Geometry check sheet. Reference: drawing and pictorial views, mm from the part's lowest x, y, z. A direction names the side the tool comes from. Round coordinates to 2 decimals unless told otherwise and drop trailing zeros. Order: outer loops, then holes, each group sorted by start corner. A loop starts at its lowest first (then second) coordinate and runs counter-clockwise, first axis right, second up.
(1) Depth check by flat-ended pin: pin 1 (1 mm diameter, centred on y = 5, z = 5, fed in from +X); pin 2 (0.6 mm diameter, centred on x = 49.5, y = 6, fed in from +Z); pin 3 (2 mm diameter, centred on x = 52, z = 5.5, fed in from +Y). Enter the tip coordinate at first touch or a pass-through.
(2) Tool access check on the marked faces 1, 2 and 3. Record the directions out of +Z, -Z, +X, -X, +Y, -Y that give a thin tool (end or side, any length) a straight path to the whole face; none if there is none.
(3) Sectioned sample at B-B, the plane z = 4.2. Enter the section's corners in (x, y), and give its area (3 significant figures).
(4) Thickness scan on probe 1 along X at (y, z) = (1.75, 0.35); probe 2 along Z at (x, y) = (70, 0.5); probe 3 along Z at (x, y) = (44, 1.5). Record the ranges inside material, lowest first.
(5) Sectioned sample at A-A, the plane y = 3. Enter the section's corners in (x, z).
(6) Sectioned sample at C-C, the plane x = 66. Enter the section's corners in (y, z).
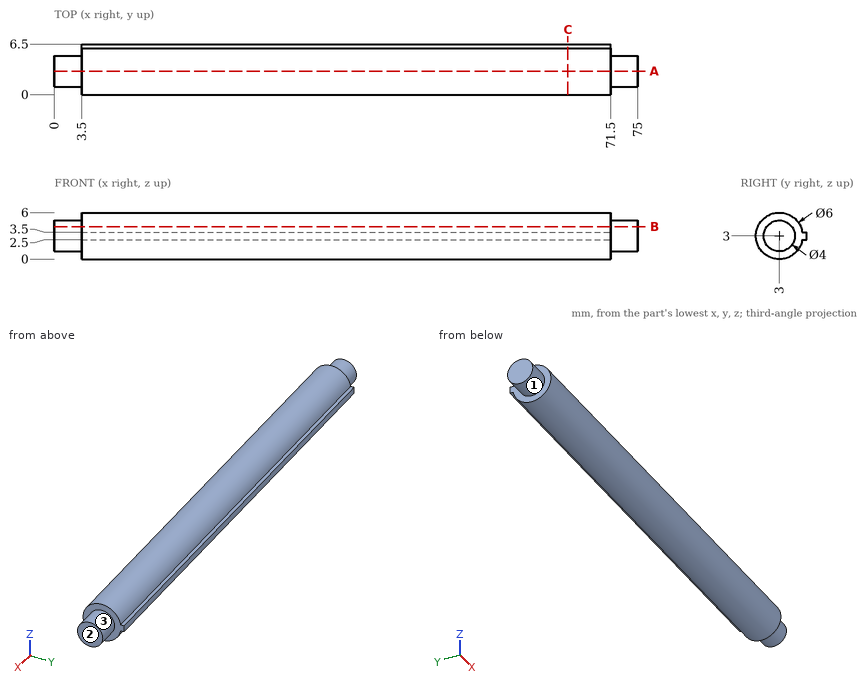
Derived:
1. pin 1: stops at x = 71.5
1. pin 2: stops at z = 4.31
1. pin 3: stops at y = 5.6
2. face 1: -X
2. face 2: +Z, -Z, +X, +Y, -Y
2. face 3: +X
3. outline: (0, 1.4) - (3.5, 1.4) - (3.5, 0.25) - (71.5, 0.25) - (71.5, 1.4) - (75, 1.4) - (75, 4.6) - (71.5, 4.6) - (71.5, 5.75) - (3.5, 5.75) - (3.5, 4.6) - (0, 4.6) - close
3. area: 396 mm2
4. probe 1: x = 3.5 to 71.5
4. probe 2: z = 1.34 to 4.66
4. probe 3: z = 0.4 to 5.6
5. outline: (0, 1) - (3.5, 1) - (3.5, 0) - (71.5, 0) - (71.5, 1) - (75, 1) - (75, 5) - (71.5, 5) - (71.5, 6) - (3.5, 6) - (3.5, 5) - (0, 5) - close
6. outline: (5.96, 2.5) - (6.5, 2.5) - (6.5, 3.5) - (5.96, 3.5) arc R3 ccw (long way) to start
